For this review, use the dimensioned drawing (mm, ordinates from the lowest corner) and the shaded views. A direction names the side the tool comes from. Coordinates: 2 decimals unless noted, no trailing zeros. Loops run counter-clockwise (first coordinate to the right, second up) from the corner with the lowest first, then second, coordinate; pieces in that order, holes last.
1. Machinability: for the marked faces 4, 5, 6 and 7, which of the approach directions +Z, -Z, +X, -X, +Y, -Y give a long, thin tool a straight path to every point of the face, cutting with its end or side? Answer none if there is none.
2. Clearance check with flat-ended pins moving along their axes: P1, Ø3, axis at y = 4.5, z = 4, coming from the +X side (3 decimals); P2, Ø1.8, axis at x = 14, z = 3.5, coming from the -Y side (3 decimals); P3, Ø2, axis at x = 3.5, y = 9.5, coming from the -Z side. State where each tip first meets the part, or that it passes through.
3. Take a section at B-B, the plane z = 2. State the section outline as (x, y) points (3 decimals).
4. To check wall thickness, follow probe 1 along Y at (x, z) = (9.5, 0.3); probe 2 along X at (y, z) = (8.75, 3.75) (3 decimals); probe 3 along Y at (x, z) = (17, 2.75) (3 decimals). State the ranges of each line that lie inside material, in increasing order.
5. Take a section at A-A, the plane y = 9.5. State the section outline as (x, z) points (3 decimals).
6. Take a section at D-D, the plane y = 16.5. State the section outline as (x, z) points (3 decimals).
7. Mouldability with a two-part tool opening along Y and no side actions: class the marked faces 1, 2 and 3 as pulls with the +Y half, pulls with the -Y half, needs draft (parallel to the pull), parting line crosses it, or undercut.
8. Take a section at C-C, the plane x = 5.5. State the section outline as (y, z) points (3 decimals), then the cut area to 3 significant figures.
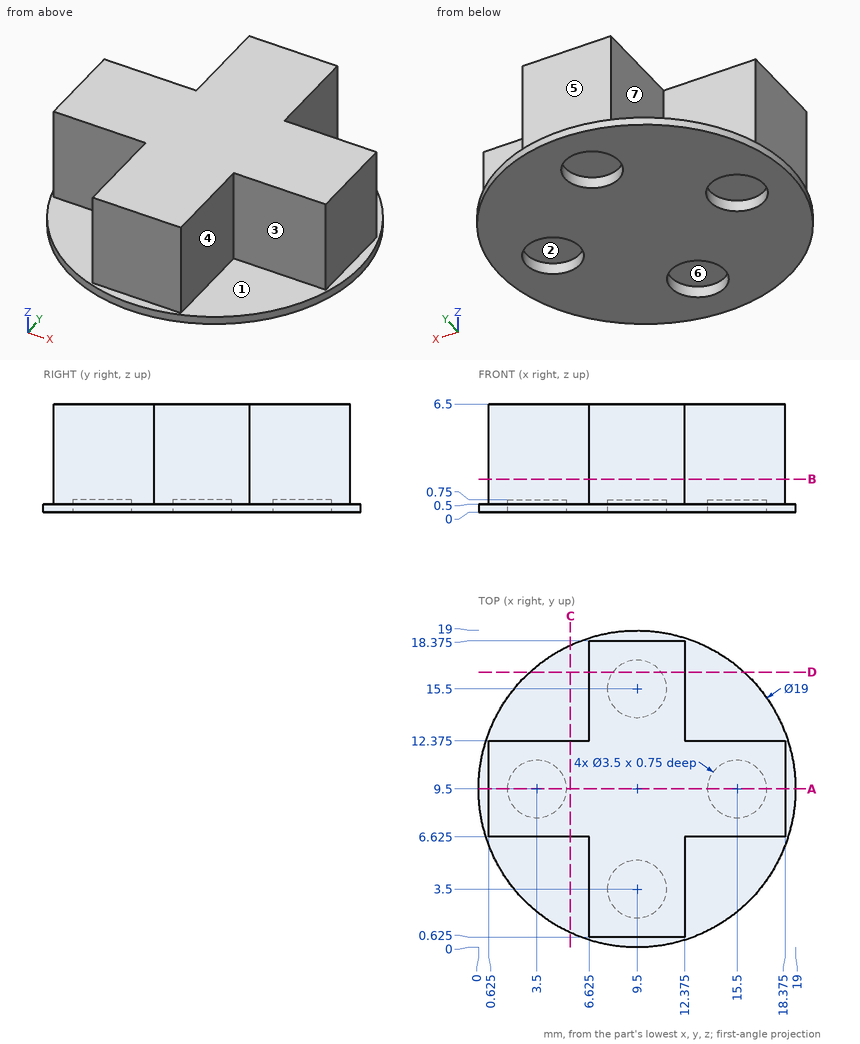
Results list:
1. face 4: +Z, +X, -Y
1. face 5: +Z, +X, -X, +Y
1. face 6: -Z
1. face 7: +Z, -X, +Y
2. P1: stops at x = 12.375
2. P2: stops at y = 6.625
2. P3: stops at z = 0.75
3. outline: (0.625, 6.625) - (6.625, 6.625) - (6.625, 0.625) - (12.375, 0.625) - (12.375, 6.625) - (18.375, 6.625) - (18.375, 12.375) - (12.375, 12.375) - (12.375, 18.375) - (6.625, 18.375) - (6.625, 12.375) - (0.625, 12.375) - close
4. probe 1: y = 0 to 1.75, 5.25 to 13.75, 17.25 to 19
4. probe 2: x = 0.625 to 18.375
4. probe 3: y = 6.625 to 12.375
5. outline: (0, 0) - (1.75, 0) - (1.75, 0.75) - (5.25, 0.75) - (5.25, 0) - (13.75, 0) - (13.75, 0.75) - (17.25, 0.75) - (17.25, 0) - (19, 0) - (19, 0.5) - (18.375, 0.5) - (18.375, 6.5) - (0.625, 6.5) - (0.625, 0.5) - (0, 0.5) - close
6. outline: (3.077, 0) - (8.064, 0) - (8.064, 0.75) - (10.936, 0.75) - (10.936, 0) - (15.923, 0) - (15.923, 0.5) - (12.375, 0.5) - (12.375, 6.5) - (6.625, 6.5) - (6.625, 0.5) - (3.077, 0.5) - close
7. face 1: needs draft
7. face 2: undercut
7. face 3: pulls with the -Y half
8. outline: (0.883, 0) - (18.117, 0) - (18.117, 0.5) - (12.375, 0.5) - (12.375, 6.5) - (6.625, 6.5) - (6.625, 0.5) - (0.883, 0.5) - close
8. area: 43.1 mm2
